Answer from the drawing. Dimensions are ordinates in mm from the lowest x, y and z of the part. A direction names the side the tool comes from. Coordinates: 2 decimals unless noted, no trailing zeros. Loops run counter-clockwise (first coordinate to the right, second up) from the corner with the lowest first, then second, coordinate; pieces in that order, holes last. Notation, with made-up numbers: (4.5, 31) - (8.5, 31) arc R20 cw to (8.5, 39) - close; hole circle Ø5 at (-2.75, 67.25). An arc over 180 degrees is marked (long way). Write each question's results on one line, items separated by ' | '. Start each with the question number.
1. A cutting plane is placed at D-D on y = 13. Determine the outline of the cut face in (x, z), then the cut area to 3 significant figures.
2. A cutting plane is placed at A-A on x = 21. Determine the outline of the cut face in (y, z), then the cut area to 3 significant figures.
3. Which of the six approach directions +Z, -Z, +X, -X, +Y, -Y give full straight-line access (tool end or side, diameter ignored) to the marked faces 1 and 2?
4. Find the intervals of material crossed by line 1 along Y through (x, z) = (36.5, 36.35); line 2 along Y through (x, z) = (5, 35); line 3 along Z through (x, y) = (37, 14), in increasing order. Write a range as [from, to].
5. A cutting plane is placed at C-C on z = 54. Determine the outline of the cut face in (x, y), then the cut area to 3 significant figures.
6. Each of these flat-tipped pins is pushed along its axis until it touches: P1, Ø1.5, axis at x = 36, y = 6, coming from the +Z side; P2, Ø3, axis at x = 26, y = 34, coming from the +Z side. Where does it stop, or does it pass through?
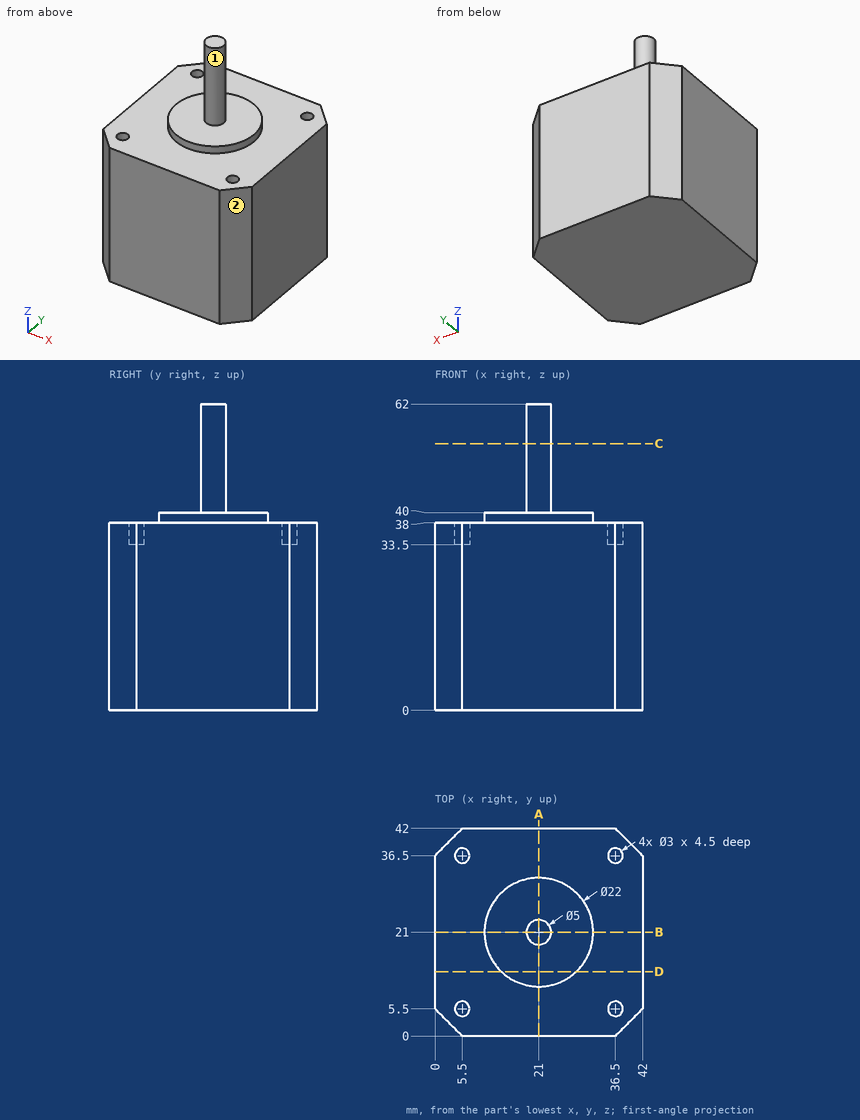
Values:
1) outline: (0, 0) - (42, 0) - (42, 38) - (28.55, 38) - (28.55, 40) - (13.45, 40) - (13.45, 38) - (0, 38) - close | area: 1,630 mm^2
2) outline: (0, 0) - (42, 0) - (42, 38) - (32, 38) - (32, 40) - (23.5, 40) - (23.5, 62) - (18.5, 62) - (18.5, 40) - (10, 40) - (10, 38) - (0, 38) - close | area: 1,750 mm^2
3) face 1: +Z | face 2: +Z, -Z, +X, -Y
4) line 1: [0, 4], [7, 35], [38, 42] | line 2: [0.5, 4.09], [6.91, 35.09], [37.91, 41.5] | line 3: [0, 38]
5) outline: circle Ø5 at (21, 21) | area: 19.6 mm^2
6) P1: z = 33.5 | P2: z = 38
